from build123d import *

# Parameters (mm, degrees)
SKETCH2_W           = 100
SKETCH2_H           = 105
BOSS_EXTRUDE1_DEPTH = 10
CUT_EXTRUDE1_REACH  = 75.186
SKETCH5_R           = 15
SKETCH5_R_2         = 5
CUT_EXTRUDE2_REACH  = 75.186
SKETCH6_W           = 22.5
SKETCH6_H           = 12.5


with BuildPart() as part:
    # Sketch2 → Boss-Extrude1 (new body)
    with BuildSketch(Plane(origin=(0, 0, 0), x_dir=(1, 0, 0), z_dir=(0, 1, 0))):
        Rectangle(SKETCH2_W, SKETCH2_H)
    extrude(amount=BOSS_EXTRUDE1_DEPTH)

    # Sketch5 → Cut-Extrude1 (cut, up to next)
    with BuildSketch(Plane.XZ, mode=Mode.PRIVATE) as cut_extrude1_sk1:
        with Locations(Location((-16.005435425, 31.5, 0), (0, 0, 270))):
            Circle(SKETCH5_R)
    cut_extrude1_tool1 = extrude(cut_extrude1_sk1.sketch, amount=-CUT_EXTRUDE1_REACH, mode=Mode.PRIVATE) & part.part
    # Sketch5 → Cut-Extrude1 (cut, up to next)
    with BuildSketch(Plane.XZ, mode=Mode.PRIVATE) as cut_extrude1_sk2:
        with Locations(Location((-39, 0, 0), (0, 0, 270))):
            Circle(SKETCH5_R_2)
    cut_extrude1_tool2 = extrude(cut_extrude1_sk2.sketch, amount=-CUT_EXTRUDE1_REACH, mode=Mode.PRIVATE) & part.part
    cut_extrude1_1 = cut_extrude1_tool1.solids().sort_by_distance((-16.005435, 0, 31.5))[0]
    add(cut_extrude1_1, mode=Mode.SUBTRACT)
    cut_extrude1_2 = cut_extrude1_tool2.solids().sort_by_distance((-39, 0, 0))[0]
    add(cut_extrude1_2, mode=Mode.SUBTRACT)
    cut_extrude1 = cut_extrude1_1 + cut_extrude1_2  # Cut-Extrude1 as one shape, for the pattern or mirror that repeats it

    # Mirror1: Cut-Extrude1 across plane
    add(cut_extrude1.mirror(Plane.XY), mode=Mode.SUBTRACT)

    # Sketch6 → Cut-Extrude2 (cut, up to next)
    with BuildSketch(Plane.XZ, mode=Mode.PRIVATE) as cut_extrude2_sk1:
        with Locations((-33.75, 0)):
            Rectangle(SKETCH6_W, SKETCH6_H)
    cut_extrude2_tool1 = extrude(cut_extrude2_sk1.sketch, amount=-CUT_EXTRUDE2_REACH, mode=Mode.PRIVATE) & part.part
    add(cut_extrude2_tool1.solids().sort_by_distance((-33.75, 0, 0))[0], mode=Mode.SUBTRACT)


solid = part.part
Input: part model. Units: mm. Frame: model coordinates. A direction names the side the tool comes from. Give positions to 0.01 mm unless a question says otherwise; leave off trailing zeros. Order: outer loops, then holes, each group sorted by start corner. A loop starts at its lowest first (then second) coordinate and runs counter-clockwise, first axis right, second up. Notation, with made-up numbers: (78.5, 29.25) - (115.5, 29.25) arc R27 cw to (115.5, 67.25) - close; hole circle Ø7 at (62, 87.5). An arc over 180 degrees is marked (long way). Answer as a JSON object with one key per item and string values. Group by question number.
Q1. Set-up query: faces 4 (the face through (-1, 10, -1)), 5 (the face through (-22.5, 5, 0)). Return all of +Z, -Z, +X, -X, +Y, -Y with unobstructed straight access to the full face (end or side cutting, diameter ignored); none if empty.
Q2. Cut plane C-C, the plane y = 6.5. Output: boundary loops of the cut face in (x, z), then the cut area to 3 significant figures.
Q3. Line query: probe 1 along Z at (x, y) = (-34, 2.75); probe 2 along X at (y, z) = (7.75, -31.5); probe 3 along Z at (x, y) = (-23, 7.25). Output: solid intervals per line, ascending.
Q4. Cut plane A-A, the plane x = -14. Output: boundary loops of the cut face in (y, z).
Q5. Cut plane D-D, the plane z = -40. Output: boundary loops of the cut face in (x, y).
Q6. Cut plane B-B, the plane z = 31.5. Output: boundary loops of the cut face in (x, y), then the cut area to 3 significant figures.
Q7. Mould query, pull axis Z, two halves, no side actions, for faces 1 (the face through (-45, 5, 0)), 2 (the face through (-1, 5, 52.5)), 3 (the face through (-50, 5, 1)). Classes: pulls with the +Z half, pulls with the -Z half, needs draft (parallel to the pull), parting line crosses it, or undercut.
Results:
{
 "1": {"face 4": "+Z, -Z, +X, -X, +Y", "face 5": "+Y, -Y"},
 "2": {"outline": "(-50, -52.5) - (50, -52.5) - (50, 52.5) - (-50, 52.5) - close; hole (-45, -6.25) - (-22.5, -6.25) - (-22.5, 6.25) - (-45, 6.25) - close; hole circle Ø30 at (-16.01, -31.5); hole circle Ø30 at (-16.01, 31.5)", "area": "8,810 mm^2"},
 "3": {"probe 1": "-52.5 to -6.25, 6.25 to 52.5", "probe 2": "-50 to -31.01, -1.01 to 50", "probe 3": "-52.5 to -44.77, -18.23 to -6.25, 6.25 to 18.23, 44.77 to 52.5"},
 "4": {"outline": "(0, -52.5) - (10, -52.5) - (10, -46.37) - (0, -46.37) - close; (0, -16.63) - (10, -16.63) - (10, 16.63) - (0, 16.63) - close; (0, 46.37) - (10, 46.37) - (10, 52.5) - (0, 52.5) - close"},
 "5": {"outline": "(-50, 0) - (-28.36, 0) - (-28.36, 10) - (-50, 10) - close; (-3.65, 0) - (50, 0) - (50, 10) - (-3.65, 10) - close"},
 "6": {"outline": "(-50, 0) - (-31.01, 0) - (-31.01, 10) - (-50, 10) - close; (-1.01, 0) - (50, 0) - (50, 10) - (-1.01, 10) - close", "area": "700 mm^2"},
 "7": {"face 1": "undercut", "face 2": "pulls with the +Z half", "face 3": "needs draft"}
}
